For this review, use the dimensioned drawing (mm, ordinates from the lowest corner) and the shaded views. Coordinates: 2 decimals unless noted, no trailing zeros. Loops run counter-clockwise (first coordinate to the right, second up) from the corner with the lowest first, then second, coordinate; pieces in that order, holes last. Notation, with made-up numbers: (-19, 85.5) - (40, 85.5) arc R12 ccw to (40, 91.5) - close; hole circle Ø4 at (12.5, 68.5). An arc over 180 degrees is marked (long way). Return JSON: item names as keys, results as strings. Group by question number.
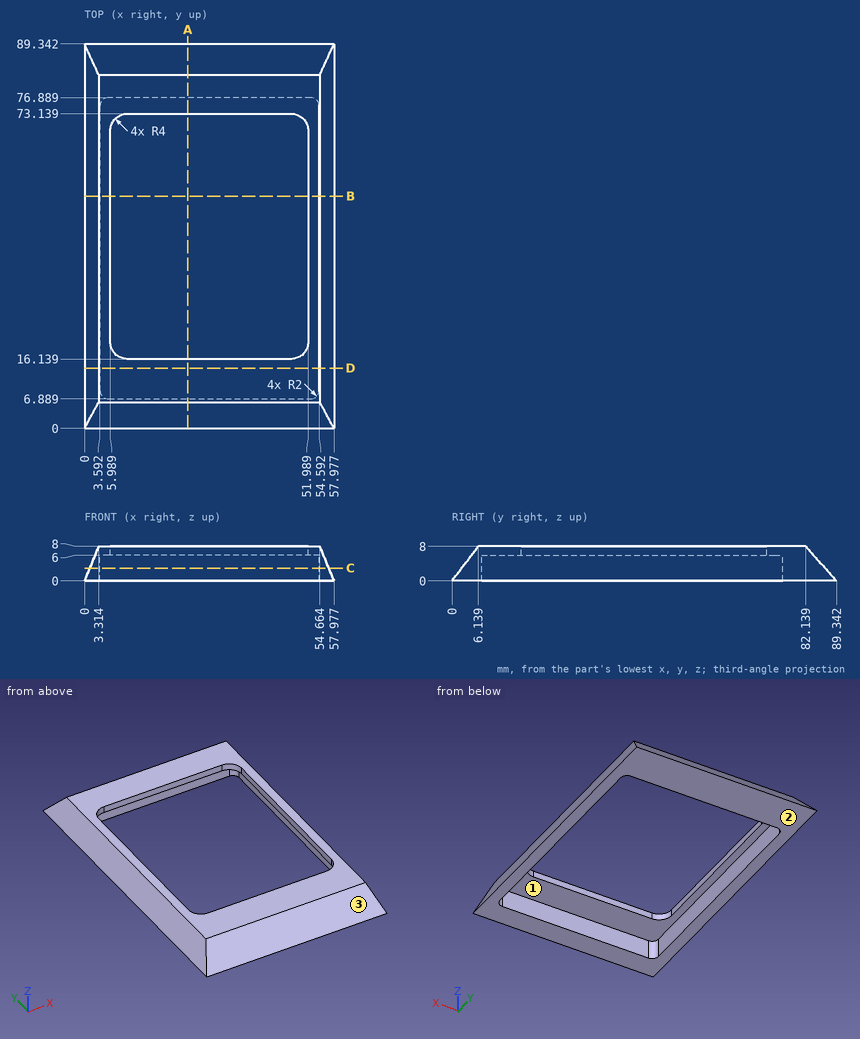
Item 1: To check wall thickness, follow line 1 (Z direction, x = 4.5, y = 13); line 2 (Y direction, x = 42, z = 1) (1 decimal); line 3 (X direction, y = 37, z = 7.25) (1 decimal). State the ranges of each line that lie inside material, in increasing order. Write a range as from..to.
Item 2: Add section A-A (x = 24). State the section outline as (y, z) points, then the cut area to 3 significant figures.
Item 3: Add section D-D (y = 14). State the section outline as (x, z) points, then the cut area to 3 significant figures.
Item 4: Add section B-B (y = 54). State the section outline as (x, z) points.
Item 5: Add section C-C (z = 3). State the section outline as (x, y) points (1 decimal).
Item 6: Draft analysis for pull direction Y (two halves, no side actions). For the marked faces 1, 2 and 3, state which applies: pulls with the +Y half, pulls with the -Y half, needs draft (parallel to the pull), parting line crosses it, or undercut.
Item 7: For P1, Ø1, axis at x = 21.5, z = 7, coming from the +Y side; P2, Ø3, axis at y = 35.5, z = 3, coming from the -X side; P3, Ø1.8, axis at y = 47.5, z = 2.5, coming from the +X side (1 decimal), all flat-tipped, find the tip position at first contact; note any pin that passes through.
Answers below:
{
 "1": {"line 1": "z = 6..8", "line 2": "y = 0.8..6.9, 76.9..88.4", "line 3": "x = 3..6, 52..55"},
 "2": {"outline": "(0, 0) - (6.89, 0) - (6.89, 6) - (16.14, 6) - (16.14, 8) - (6.14, 8) - close; (73.14, 6) - (76.89, 6) - (76.89, 0) - (89.34, 0) - (82.14, 8) - (73.14, 8) - close", "area": "127 mm^2"},
 "3": {"outline": "(0, 0) - (3.59, 0) - (3.59, 6) - (54.59, 6) - (54.59, 0) - (57.98, 0) - (54.66, 8) - (3.31, 8) - close", "area": "131 mm^2"},
 "4": {"outline": "(0, 0) - (3.59, 0) - (3.59, 6) - (5.99, 6) - (5.99, 8) - (3.31, 8) - close; (51.99, 6) - (54.59, 6) - (54.59, 0) - (57.98, 0) - (54.66, 8) - (51.99, 8) - close"},
 "5": {"outline": "(1.2, 2.3) - (56.7, 2.3) - (56.7, 86.6) - (1.2, 86.6) - close; hole (3.6, 8.9) arc R2 ccw to (5.6, 6.9) - (52.6, 6.9) arc R2 ccw to (54.6, 8.9) - (54.6, 74.9) arc R2 ccw to (52.6, 76.9) - (5.6, 76.9) arc R2 ccw to (3.6, 74.9) - close"},
 "6": {"face 1": "undercut", "face 2": "needs draft", "face 3": "pulls with the -Y half"},
 "7": {"P1": "stops at y = 83.49", "P2": "stops at x = 0.62", "P3": "stops at x = 57.3"}
}
